Part model, mm, in its own coordinate system. Face numbers are marked on the shaded views. A direction names the side the tool comes from. Coordinates: 2 decimals unless noted, no trailing zeros. Loops run counter-clockwise (first coordinate to the right, second up) from the corner with the lowest first, then second, coordinate; pieces in that order, holes last. Notation, with made-up numbers: M -2,-25 L 32,-25 A19 ccw 32,-14 Z; hole C 84,9 d2. An arc over 180 degrees is marked long. Answer as a JSON object with one key per item and string values. Group by question number.
1. Saw through at C-C on x = -31. Count the separate pieces of the cut face and the enclosed holes in it, then the cut area to 3 significant figures.
2. 3-axis set-ups, long thin cutter, end or side, ignore diameter. For the marked faces 1 and 2: which of +Z, -Z, +X, -X, +Y, -Y reach the whole face in a straight line?
3. Drop flat-ended pins along their axis: pin 1 Ø3.5 at (x, y) = (-21, -15.5) entering from -Z; pin 2 Ø1.1 at (x, y) = (-13, 20) entering from +Z; pin 3 Ø1 at (x, z) = (-27.5, 0.5) entering from +Y; pin 4 Ø0.8 at (x, z) = (-20.5, 19.5) entering from +Y. Give the stop position or say it passes through.
4. Mould opens along Y. For the marked faces 3, 4, 5 and 6 say: released by +Y, released by -Y, zero draft, split by the parting line, or undercut.
5. Saw through at A-A on z = 14. Write the cut outline in (x, y).
6. Drill centre lines: L1, parallel to Y at x = -39.5, z = -5; L2, parallel to Y at x = -14, z = -4; L3, parallel to Y at x = -36, z = -15.5. Where is each one in solid material? Low to high.
from build123d import *

# Parameters (mm, degrees)
EXTRUDE_1_DEPTH = 50


with BuildPart() as part:
    # 草图1 → 凸台-拉伸1 (new body)
    with BuildSketch(Plane(origin=(0, 0, 0), x_dir=(0, 0, -1), z_dir=(1, 0, 0))):
        with BuildLine():
            Line((4.82004008, 19.27995992), (3.82004008, 19.27995992))
            Line((3.82004008, 19.27995992), (3.82004008, 15.77995992))
            Line((3.82004008, 15.77995992), (6.73639159, 15.77995992))
            Line((6.73639159, 15.77995992), (6.73639159, 18.02995992))
            Line((6.73639159, 18.02995992), (10.02004008, 18.02995992))
            Line((10.02004008, 18.02995992), (10.02004008, 12.70128026))
            Line((10.02004008, 12.70128026), (5.19871974, 7.87995992))
            Line((5.19871974, 7.87995992), (-5.75863958, 7.87995992))
            Line((-5.75863958, 7.87995992), (-10.57995992, 12.70128026))
            Line((-10.57995992, 12.70128026), (-10.57995992, 18.02995992))
            Line((-10.57995992, 18.02995992), (-7.29631143, 18.02995992))
            Line((-7.29631143, 18.02995992), (-7.29631143, 15.77995992))
            Line((-7.29631143, 15.77995992), (-4.37995992, 15.77995992))
            Line((-4.37995992, 15.77995992), (-4.37995992, 19.27995992))
            Line((-4.37995992, 19.27995992), (-5.37995992, 19.27995992))
            Line((-5.37995992, 19.27995992), (-5.37995992, 20.27995992))
            Line((-5.37995992, 20.27995992), (-15.77995992, 20.27995992))
            ThreePointArc((-15.77995992, 20.27995992), (-18.961940435, 18.961940435), (-20.27995992, 15.77995992))
            Line((-20.27995992, 15.77995992), (-20.27995992, 5.37995992))
            Line((-20.27995992, 5.37995992), (-19.27995992, 5.37995992))
            Line((-19.27995992, 5.37995992), (-19.27995992, 4.37995992))
            Line((-19.27995992, 4.37995992), (-15.77995992, 4.37995992))
            Line((-15.77995992, 4.37995992), (-15.77995992, 7.29631143))
            Line((-15.77995992, 7.29631143), (-18.02995992, 7.29631143))
            Line((-18.02995992, 7.29631143), (-18.02995992, 10.57995992))
            Line((-18.02995992, 10.57995992), (-12.70128026, 10.57995992))
            Line((-12.70128026, 10.57995992), (-7.87995992, 5.75863958))
            Line((-7.87995992, 5.75863958), (-7.87995992, -5.19871974))
            Line((-7.87995992, -5.19871974), (-12.70128026, -10.02004008))
            Line((-12.70128026, -10.02004008), (-18.02995992, -10.02004008))
            Line((-18.02995992, -10.02004008), (-18.02995992, -6.73639159))
            Line((-18.02995992, -6.73639159), (-15.77995992, -6.73639159))
            Line((-15.77995992, -6.73639159), (-15.77995992, -3.82004008))
            Line((-15.77995992, -3.82004008), (-19.27995992, -3.82004008))
            Line((-19.27995992, -3.82004008), (-19.27995992, -4.82004008))
            Line((-19.27995992, -4.82004008), (-20.27995992, -4.82004008))
            Line((-20.27995992, -4.82004008), (-20.27995992, -15.22004008))
            ThreePointArc((-20.27995992, -15.22004008), (-18.961940435, -18.402020595), (-15.77995992, -19.72004008))
            Line((-15.77995992, -19.72004008), (-5.37995992, -19.72004008))
            Line((-5.37995992, -19.72004008), (-5.37995992, -18.72004008))
            Line((-5.37995992, -18.72004008), (-4.37995992, -18.72004008))
            Line((-4.37995992, -18.72004008), (-4.37995992, -15.22004008))
            Line((-4.37995992, -15.22004008), (-7.29631143, -15.22004008))
            Line((-7.29631143, -15.22004008), (-7.29631143, -17.47004008))
            Line((-7.29631143, -17.47004008), (-10.57995992, -17.47004008))
            Line((-10.57995992, -17.47004008), (-10.57995992, -12.14136042))
            Line((-10.57995992, -12.14136042), (-5.75863958, -7.32004008))
            Line((-5.75863958, -7.32004008), (5.19871974, -7.32004008))
            Line((5.19871974, -7.32004008), (10.02004008, -12.14136042))
            Line((10.02004008, -12.14136042), (10.02004008, -17.47004008))
            Line((10.02004008, -17.47004008), (6.73639159, -17.47004008))
            Line((6.73639159, -17.47004008), (6.73639159, -15.22004008))
            Line((6.73639159, -15.22004008), (3.82004008, -15.22004008))
            Line((3.82004008, -15.22004008), (3.82004008, -18.72004008))
            Line((3.82004008, -18.72004008), (4.82004008, -18.72004008))
            Line((4.82004008, -18.72004008), (4.82004008, -19.72004008))
            Line((4.82004008, -19.72004008), (15.22004008, -19.72004008))
            ThreePointArc((15.22004008, -19.72004008), (18.402020595, -18.402020595), (19.72004008, -15.22004008))
            Line((19.72004008, -15.22004008), (19.72004008, -4.82004008))
            Line((19.72004008, -4.82004008), (18.72004008, -4.82004008))
            Line((18.72004008, -4.82004008), (18.72004008, -3.82004008))
            Line((18.72004008, -3.82004008), (15.22004008, -3.82004008))
            Line((15.22004008, -3.82004008), (15.22004008, -6.73639159))
            Line((15.22004008, -6.73639159), (17.47004008, -6.73639159))
            Line((17.47004008, -6.73639159), (17.47004008, -10.02004008))
            Line((17.47004008, -10.02004008), (12.14136042, -10.02004008))
            Line((12.14136042, -10.02004008), (7.32004008, -5.19871974))
            Line((7.32004008, -5.19871974), (7.32004008, 5.75863958))
            Line((7.32004008, 5.75863958), (12.14136042, 10.57995992))
            Line((12.14136042, 10.57995992), (17.47004008, 10.57995992))
            Line((17.47004008, 10.57995992), (17.47004008, 7.29631143))
            Line((17.47004008, 7.29631143), (15.22004008, 7.29631143))
            Line((15.22004008, 7.29631143), (15.22004008, 4.37995992))
            Line((15.22004008, 4.37995992), (18.72004008, 4.37995992))
            Line((18.72004008, 4.37995992), (18.72004008, 5.37995992))
            Line((18.72004008, 5.37995992), (19.72004008, 5.37995992))
            Line((19.72004008, 5.37995992), (19.72004008, 15.77995992))
            ThreePointArc((19.72004008, 15.77995992), (18.402020595, 18.961940435), (15.22004008, 20.27995992))
            Line((15.22004008, 20.27995992), (4.82004008, 20.27995992))
            Line((4.82004008, 20.27995992), (4.82004008, 19.27995992))
        make_face()
        with BuildLine():
            Line((-13.07995992, -17.72004008), (-17.27995992, -17.72004008))
            ThreePointArc((-17.27995992, -17.72004008), (-17.987066701, -17.427146861), (-18.27995992, -16.72004008))
            Line((-18.27995992, -16.72004008), (-18.27995992, -12.52004008))
            ThreePointArc((-18.27995992, -12.52004008), (-17.987066701, -11.812933299), (-17.27995992, -11.52004008))
            Line((-17.27995992, -11.52004008), (-13.07995992, -11.52004008))
            ThreePointArc((-13.07995992, -11.52004008), (-12.372853139, -11.812933299), (-12.07995992, -12.52004008))
            Line((-12.07995992, -12.52004008), (-12.07995992, -16.72004008))
            ThreePointArc((-12.07995992, -16.72004008), (-12.372853139, -17.427146861), (-13.07995992, -17.72004008))
        make_face(mode=Mode.SUBTRACT)
        with BuildLine():
            Line((-17.27995992, 18.27995992), (-13.07995992, 18.27995992))
            ThreePointArc((-13.07995992, 18.27995992), (-12.372853139, 17.987066701), (-12.07995992, 17.27995992))
            Line((-12.07995992, 17.27995992), (-12.07995992, 13.07995992))
            ThreePointArc((-12.07995992, 13.07995992), (-12.372853139, 12.372853139), (-13.07995992, 12.07995992))
            Line((-13.07995992, 12.07995992), (-17.27995992, 12.07995992))
            ThreePointArc((-17.27995992, 12.07995992), (-17.987066701, 12.372853139), (-18.27995992, 13.07995992))
            Line((-18.27995992, 13.07995992), (-18.27995992, 17.27995992))
            ThreePointArc((-18.27995992, 17.27995992), (-17.987066701, 17.987066701), (-17.27995992, 18.27995992))
        make_face(mode=Mode.SUBTRACT)
        with BuildLine():
            Line((16.72004008, 12.07995992), (12.52004008, 12.07995992))
            ThreePointArc((12.52004008, 12.07995992), (11.812933299, 12.372853139), (11.52004008, 13.07995992))
            Line((11.52004008, 13.07995992), (11.52004008, 17.27995992))
            ThreePointArc((11.52004008, 17.27995992), (11.812933299, 17.987066701), (12.52004008, 18.27995992))
            Line((12.52004008, 18.27995992), (16.72004008, 18.27995992))
            ThreePointArc((16.72004008, 18.27995992), (17.427146861, 17.987066701), (17.72004008, 17.27995992))
            Line((17.72004008, 17.27995992), (17.72004008, 13.07995992))
            ThreePointArc((17.72004008, 13.07995992), (17.427146861, 12.372853139), (16.72004008, 12.07995992))
        make_face(mode=Mode.SUBTRACT)
        with BuildLine():
            Line((3.75045895, -3.04335217), (3.04335217, -3.75045895))
            Line((3.04335217, -3.75045895), (1.74451108, -2.45161786))
            ThreePointArc((1.74451108, -2.45161786), (-0.27995992, -3.12004008), (-2.30443092, -2.45161786))
            Line((-2.30443092, -2.45161786), (-3.60327201, -3.75045895))
            Line((-3.60327201, -3.75045895), (-4.31037879, -3.04335217))
            Line((-4.31037879, -3.04335217), (-3.0115377, -1.74451108))
            ThreePointArc((-3.0115377, -1.74451108), (-3.67995992, 0.27995992), (-3.0115377, 2.30443092))
            Line((-3.0115377, 2.30443092), (-4.31037879, 3.60327201))
            Line((-4.31037879, 3.60327201), (-3.60327201, 4.31037879))
            Line((-3.60327201, 4.31037879), (-2.30443092, 3.0115377))
            ThreePointArc((-2.30443092, 3.0115377), (-0.27995992, 3.67995992), (1.74451108, 3.0115377))
            Line((1.74451108, 3.0115377), (3.04335217, 4.31037879))
            Line((3.04335217, 4.31037879), (3.75045895, 3.60327201))
            Line((3.75045895, 3.60327201), (2.45161786, 2.30443092))
            ThreePointArc((2.45161786, 2.30443092), (3.12004008, 0.27995992), (2.45161786, -1.74451108))
            Line((2.45161786, -1.74451108), (3.75045895, -3.04335217))
        make_face(mode=Mode.SUBTRACT)
        with BuildLine():
            Line((17.72004008, -12.52004008), (17.72004008, -16.72004008))
            ThreePointArc((17.72004008, -16.72004008), (17.427146861, -17.427146861), (16.72004008, -17.72004008))
            Line((16.72004008, -17.72004008), (12.52004008, -17.72004008))
            ThreePointArc((12.52004008, -17.72004008), (11.812933299, -17.427146861), (11.52004008, -16.72004008))
            Line((11.52004008, -16.72004008), (11.52004008, -12.52004008))
            ThreePointArc((11.52004008, -12.52004008), (11.812933299, -11.812933299), (12.52004008, -11.52004008))
            Line((12.52004008, -11.52004008), (16.72004008, -11.52004008))
            ThreePointArc((16.72004008, -11.52004008), (17.427146861, -11.812933299), (17.72004008, -12.52004008))
        make_face(mode=Mode.SUBTRACT)
    extrude(amount=-EXTRUDE_1_DEPTH)


solid = part.part
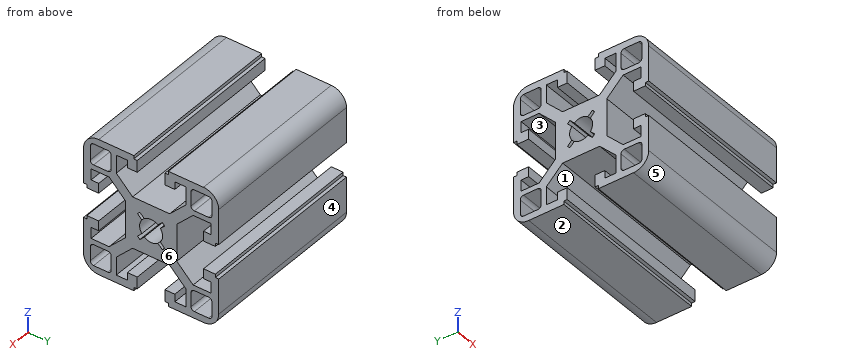
Outcome:
{
 "1": {"separate pieces": "1", "enclosed holes": "5", "area": "616 mm²"},
 "2": {"face 1": "+X, -X", "face 2": "-Z, +X, -X, +Y, -Y"},
 "3": {"pin 1": "stops at z = -19.72", "pin 2": "stops at z = 18.38", "pin 3": "stops at y = 7.88", "pin 4": "stops at y = 18.82"},
 "4": {"face 3": "undercut", "face 4": "released by +Y", "face 5": "released by -Y", "face 6": "zero draft"},
 "5": {"outline": "M -50,-19.72 L 0,-19.72 L 0,-17.72 L -50,-17.72 Z; M -50,-11.52 L 0,-11.52 L 0,-10.02 L -50,-10.02 Z; M -50,10.58 L 0,10.58 L 0,12.08 L -50,12.08 Z; M -50,18.28 L 0,18.28 L 0,20.28 L -50,20.28 Z"},
 "6": {"L1": "y = -19.72 to -15.22, -7.32 to 7.88, 15.78 to 20.28", "L2": "y = -18.72 to -15.22, -7.32 to 7.88, 15.78 to 19.28", "L3": "y = -19.71 to -17.72, -11.52 to -10.02, -6.74 to -3.82, 4.38 to 7.3, 10.58 to 12.08, 18.28 to 20.27"}
}
